from build123d import *

# Parameters (mm, degrees)
BOSS_EXTRUDE1_DEPTH = 50.8
SKETCH2_R           = 12.7
CUT_EXTRUDE1_DEPTH  = 86.09
SKETCH3_R           = 12.7
BOSS_EXTRUDE2_DEPTH = 6.35
SKETCH4_R           = 19.05
BOSS_EXTRUDE3_DEPTH = 1.27
SKETCH5_R           = 12.7
BOSS_EXTRUDE4_DEPTH = 25.4
SKETCH6_R           = 6.35
CUT_EXTRUDE2_DEPTH  = 174.99
SKETCH7_R           = 19.05
SKETCH7_R_2         = 12.7
BOSS_EXTRUDE5_DEPTH = 2.54


with BuildPart() as part:
    # Sketch1 → Boss-Extrude1 (new body)
    with BuildSketch(Plane.XY):
        with BuildLine():
            Line((42.545, 113.03), (42.545, -25.4))
            Line((42.545, -25.4), (41.275, -25.4))
            Line((41.275, -25.4), (41.275, 111.76))
            ThreePointArc((41.275, 111.76), (40.531051224, 113.556051224), (38.735, 114.3))
            Line((38.735, 114.3), (-38.735, 114.3))
            ThreePointArc((-38.735, 114.3), (-40.531051224, 113.556051224), (-41.275, 111.76))
            Line((-41.275, 111.76), (-41.275, -25.4))
            Line((-41.275, -25.4), (-42.545, -25.4))
            Line((-42.545, -25.4), (-42.545, 113.03))
            ThreePointArc((-42.545, 113.03), (-41.801051224, 114.826051224), (-40.005, 115.57))
            Line((-40.005, 115.57), (40.005, 115.57))
            ThreePointArc((40.005, 115.57), (41.801051224, 114.826051224), (42.545, 113.03))
        make_face()
    extrude(amount=BOSS_EXTRUDE1_DEPTH)

    # Sketch2 → Cut-Extrude1 (cut, through all)
    with BuildSketch(Plane.ZY.offset(42.545)):
        with Locations((25.4, 0)):
            Circle(SKETCH2_R)
    extrude(amount=-CUT_EXTRUDE1_DEPTH, mode=Mode.SUBTRACT)

    # Sketch3 → Boss-Extrude2 (add)
    with BuildSketch(Plane(origin=(0, 115.57, 0), x_dir=(1, 0, 0), z_dir=(0, 1, 0))):
        with Locations((0, -25.4)):
            Circle(SKETCH3_R)
    extrude(amount=BOSS_EXTRUDE2_DEPTH)

    # Sketch4 → Boss-Extrude3 (add)
    with BuildSketch(Plane(origin=(0, 121.92, 0), x_dir=(1, 0, 0), z_dir=(0, 1, 0))):
        with Locations((0, -25.4)):
            Circle(SKETCH4_R)
    extrude(amount=BOSS_EXTRUDE3_DEPTH)

    # Sketch5 → Boss-Extrude4 (add)
    with BuildSketch(Plane(origin=(0, 123.19, 0), x_dir=(1, 0, 0), z_dir=(0, 1, 0))):
        with Locations((0, -25.4)):
            Circle(SKETCH5_R)
    extrude(amount=BOSS_EXTRUDE4_DEPTH)

    # Sketch6 → Cut-Extrude2 (cut, through all)
    with BuildSketch(Plane(origin=(0, 148.59, 0), x_dir=(1, 0, 0), z_dir=(0, 1, 0))):
        with Locations((0, -25.4)):
            Circle(SKETCH6_R)
    extrude(amount=-CUT_EXTRUDE2_DEPTH, mode=Mode.SUBTRACT)

    # Sketch7 → Boss-Extrude5 (add)
    with BuildSketch(Plane(origin=(0, 127, 0), x_dir=(1, 0, 0), z_dir=(0, 1, 0))):
        with Locations((0, -25.4)):
            Circle(SKETCH7_R)
        with Locations((0, -25.4)):
            Circle(SKETCH7_R_2, mode=Mode.SUBTRACT)
    extrude(amount=BOSS_EXTRUDE5_DEPTH)


solid = part.part
Geometry check sheet. Reference: the model listing, model coordinates, mm. A direction names the side the tool comes from. Round coordinates to 2 decimals unless told otherwise and drop trailing zeros. Order: outer loops, then holes, each group sorted by start corner. A loop starts at its lowest first (then second) coordinate and runs counter-clockwise, first axis right, second up. Notation, with made-up numbers: (-10.5, -21.75) - (20.5, -21.75) arc R18 ccw to (20.5, -16.75) - close; hole circle Ø3 at (42, -29). An arc over 180 degrees is marked (long way). One line per question, with ' | ' between items. Start each with the question number.
(1) Thickness scan on L1, parallel to Y at x = 4.5, z = 38; L2, parallel to X at y = 90, z = 24 (3 decimals); L3, parallel to X at y = 139, z = 25. Record the ranges inside material, lowest first. Write a range as [from, to].
(2) Sectioned sample at D-D on z = 40. Record the cut outline in (x, y) (3 decimals), and give its area (3 significant figures).
(3) Release check for a two-part mould opening along Y. For faces 1 (the flat face through (-42.545, 43, 25)), 2 (the flat face through (12.4, 129.54, 29.4)), 3 (the cylindrical face through (-2.75, 118.7, 37.8)) record: released by +Y, released by -Y, zero draft, split by the parting line, or undercut.
(4) Depth check by flat-ended pin: pin 1 Ø3 at (x, z) = (-22, 39.5) entering from +Y; pin 2 Ø5 at (x, z) = (20.5, 25) entering from +Y; pin 3 Ø10 at (x, z) = (0, 25.4) entering from +Y (1 decimal); pin 4 Ø3 at (x, y) = (6.5, 129) entering from -Z. Enter the tip coordinate at first touch or a pass-through.
(5) Sectioned sample at A-A on x = 0. Record the cut outline in (y, z).
(6) Access from +Z, -Z, +X, -X, +Y, -Y to the whole of each face (thin tool, end or side, straight path). Record for faces 4 (the cylindrical face through (41.901, 0.558, 12.712)), 5 (the flat face through (12.4, 123.19, 29.4)), 6 (the flat face through (-41.275, 44, 25)), 7 (the cylindrical face through (-2.48, 128.252, 6.512)), 8 (the flat face through (42.545, 45, 25)).
(7) Sectioned sample at C-C on y = 0. Record the cut outline in (x, z) (3 decimals), and give its area (3 significant figures).
(8) Sectioned sample at B-B on y = 56. Record the cut outline in (x, z) (3 decimals).
Conclusion:
1) L1: y = [114.3, 115.57], [121.92, 123.19], [127, 129.54] | L2: x = [-42.545, -41.275], [41.275, 42.545] | L3: x = [-12.69, -6.34], [6.34, 12.69]
2) outline: (-42.545, -25.4) - (-41.275, -25.4) - (-41.275, 111.76) arc R2.54 cw to (-38.735, 114.3) - (38.735, 114.3) arc R2.54 cw to (41.275, 111.76) - (41.275, -25.4) - (42.545, -25.4) - (42.545, 113.03) arc R2.54 ccw to (40.005, 115.57) - (-40.005, 115.57) arc R2.54 ccw to (-42.545, 113.03) - close; (-12.237, 121.92) - (12.237, 121.92) - (12.237, 123.19) - (-12.237, 123.19) - close; (-12.237, 127) - (12.237, 127) - (12.237, 129.54) - (-12.237, 129.54) - close | area: 556 mm2
3) face 1: zero draft | face 2: released by +Y | face 3: undercut
4) pin 1: stops at y = 115.57 | pin 2: stops at y = 129.54 | pin 3: passes through | pin 4: stops at z = 7.02
5) outline: (114.3, 0) - (115.57, 0) - (115.57, 12.7) - (121.92, 12.7) - (121.92, 6.35) - (123.19, 6.35) - (123.19, 12.7) - (127, 12.7) - (127, 6.35) - (129.54, 6.35) - (129.54, 12.7) - (148.59, 12.7) - (148.59, 19.05) - (114.3, 19.05) - close; (114.3, 31.75) - (148.59, 31.75) - (148.59, 38.1) - (129.54, 38.1) - (129.54, 44.45) - (127, 44.45) - (127, 38.1) - (123.19, 38.1) - (123.19, 44.45) - (121.92, 44.45) - (121.92, 38.1) - (115.57, 38.1) - (115.57, 50.8) - (114.3, 50.8) - close
6) face 4: +X, -X | face 5: none | face 6: +Z, -Z, -Y | face 7: +Y | face 8: +Z, -Z, +X, +Y, -Y
7) outline: (-42.545, 0) - (-41.275, 0) - (-41.275, 12.7) - (-42.545, 12.7) - close; (-42.545, 38.1) - (-41.275, 38.1) - (-41.275, 50.8) - (-42.545, 50.8) - close; (41.275, 0) - (42.545, 0) - (42.545, 12.7) - (41.275, 12.7) - close; (41.275, 38.1) - (42.545, 38.1) - (42.545, 50.8) - (41.275, 50.8) - close | area: 64.5 mm2
8) outline: (-42.545, 0) - (-41.275, 0) - (-41.275, 50.8) - (-42.545, 50.8) - close; (41.275, 0) - (42.545, 0) - (42.545, 50.8) - (41.275, 50.8) - close
